Source: CAD feature listing. Evaluate the final solid. Frame: model axes, mm. A direction names the side the tool comes from. Give positions to 0.01 mm unless a question says otherwise; leave off trailing zeros. Loops run counter-clockwise (first coordinate to the right, second up) from the corner with the lowest first, then second, coordinate; pieces in that order, holes last. Notation, with made-up numbers: M 71.25,-29.5 L 101.25,-29.5 A6 cw 101.25,-19.5 Z; hole C 31,88.5 d3. An arc over 180 degrees is marked long. Answer in a Markdown table with one row per item.
```python
from build123d import *

# Parameters (mm, degrees)
BOX005_W        = 20
BOX005_H        = 1
BOX005_DEPTH    = 56
BOX006_W        = 20
BOX006_H        = 1
BOX006_DEPTH    = 56
BOX004_W        = 200
BOX004_H        = 1
BOX004_DEPTH    = 40
BOX002_W        = 1
BOX002_H        = 150
BOX002_DEPTH    = 56
BOX001_W        = 1
BOX001_H        = 150
BOX001_DEPTH    = 56
BOX_W           = 200
BOX_H           = 150
BOX_DEPTH       = 1
BOX003_W        = 200
BOX003_H        = 1
BOX003_DEPTH    = 56
CHAMFER_SIZE    = 2
CHAMFER001_SIZE = 2
CHAMFER002_SIZE = 2
CHAMFER003_SIZE = 2
CHAMFER004_SIZE = 2
CHAMFER005_SIZE = 2


with BuildPart() as cube005:
    # Box005 → Box005 (new body)
    with BuildSketch(Plane.XY):
        with Locations((10, 0.5)):
            Rectangle(BOX005_W, BOX005_H)
    extrude(amount=BOX005_DEPTH)


with BuildPart() as cube006:
    # Box006 → Box006 (new body)
    with BuildSketch(Plane(origin=(180, 0, 0), x_dir=(1, 0, 0), z_dir=(0, 0, 1))):
        with Locations((10, 0.5)):
            Rectangle(BOX006_W, BOX006_H)
    extrude(amount=BOX006_DEPTH)


with BuildPart() as cube004:
    # Box004 → Box004 (new body)
    with BuildSketch(Plane.XY):
        with Locations((100, 0.5)):
            Rectangle(BOX004_W, BOX004_H)
    extrude(amount=BOX004_DEPTH)


with BuildPart() as cube002:
    # Box002 → Box002 (new body)
    with BuildSketch(Plane(origin=(199, 0, 0), x_dir=(1, 0, 0), z_dir=(0, 0, 1))):
        with Locations((0.5, 75)):
            Rectangle(BOX002_W, BOX002_H)
    extrude(amount=BOX002_DEPTH)


with BuildPart() as cube001:
    # Box001 → Box001 (new body)
    with BuildSketch(Plane.XY):
        with Locations((0.5, 75)):
            Rectangle(BOX001_W, BOX001_H)
    extrude(amount=BOX001_DEPTH)


with BuildPart() as cube:
    # Box → Box (new body)
    with BuildSketch(Plane.XY):
        with Locations((100, 75)):
            Rectangle(BOX_W, BOX_H)
    extrude(amount=BOX_DEPTH)


with BuildPart() as fusion005:
    # Box003 → Box003 (new body)
    with BuildSketch(Plane(origin=(0, 149, 0), x_dir=(1, 0, 0), z_dir=(0, 0, 1))):
        with Locations((100, 0.5)):
            Rectangle(BOX003_W, BOX003_H)
    extrude(amount=BOX003_DEPTH)

    # Fusion: union Cube
    add(cube.part)

    # Fusion001: union Cube001
    add(cube001.part)

    # Fusion002: union Cube002
    add(cube002.part)

    # Fusion003: union Cube004
    add(cube004.part)

    # Chamfer
    chamfer_edges = [fusion005.edges().sort_by_distance(p)[0] for p in [
        (100, 149, 1),
    ]]
    chamfer(chamfer_edges, length=CHAMFER_SIZE)

    # Chamfer001
    chamfer001_edges = [fusion005.edges().sort_by_distance(p)[0] for p in [
        (1, 74, 1),
    ]]
    chamfer(chamfer001_edges, length=CHAMFER001_SIZE)

    # Chamfer002
    chamfer002_edges = [fusion005.edges().sort_by_distance(p)[0] for p in [
        (199, 74, 1),
    ]]
    chamfer(chamfer002_edges, length=CHAMFER002_SIZE)

    # Chamfer003
    chamfer003_edges = [fusion005.edges().sort_by_distance(p)[0] for p in [
        (1, 149, 29.5),
    ]]
    chamfer(chamfer003_edges, length=CHAMFER003_SIZE)

    # Chamfer004
    chamfer004_edges = [fusion005.edges().sort_by_distance(p)[0] for p in [
        (199, 149, 29.5),
    ]]
    chamfer(chamfer004_edges, length=CHAMFER004_SIZE)

    # Chamfer005
    chamfer005_edges = [fusion005.edges().sort_by_distance(p)[0] for p in [
        (100, 1, 1),
    ]]
    chamfer(chamfer005_edges, length=CHAMFER005_SIZE)

    # Fusion004: union Cube006
    add(cube006.part)

    # Fusion005: union Cube005
    add(cube005.part)


solid = fusion005.part
```
1) Material intervals for L1, parallel to X at y = 123, z = 10.5; L2, parallel to Y at x = 129.5, z = 18; L3, parallel to Z at x = 18, y = 82.5, sorted ascending.
Reply:
| item | result |
|---|---|
| L1 | x = 0 to 1, 199 to 200 |
| L2 | y = 0 to 1, 149 to 150 |
| L3 | z = 0 to 1 |
2) Pull-direction query (Y, two-part tool) for faces 1 (the flat face through (99, 150, 28)), 2 (the flat face through (99, 0, 21)), 3 (the flat face through (1, 73, 29)), 4 (the flat face through (199, 73, 29)); classes: released by +Y, released by -Y, zero draft, split by the parting line, or undercut.
Reply:
| item | result |
|---|---|
| face 1 | released by +Y |
| face 2 | released by -Y |
| face 3 | undercut |
| face 4 | undercut |
3) Section C-C, the plane z = 10.5. Return loops of the section in (x, y).
Reply:
| item | result |
|---|---|
| outline | M 0,0 L 200,0 L 200,150 L 0,150 Z; hole M 1,1 L 199,1 L 199,147 L 197,149 L 3,149 L 1,147 Z |
4) Section D-D, the plane x = 25.5. Return loops of the section in (y, z), then the cut area to 3 significant figures.
Reply:
| item | result |
|---|---|
| outline | M 0,0 L 150,0 L 150,56 L 149,56 L 149,3 L 147,1 L 3,1 L 1,3 L 1,40 L 0,40 Z |
| area | 248 mm² |
5) Section A-A, the plane y = 62.5. Return loops of the section in (x, z), then the cut area to 3 significant figures.
Reply:
| item | result |
|---|---|
| outline | M 0,0 L 200,0 L 200,56 L 199,56 L 199,3 L 197,1 L 3,1 L 1,3 L 1,56 L 0,56 Z |
| area | 314 mm² |
6) Section B-B, the plane z = 50. Return loops of the section in (x, y).
Reply:
| item | result |
|---|---|
| outline | M 0,0 L 20,0 L 20,1 L 1,1 L 1,147 L 3,149 L 197,149 L 199,147 L 199,1 L 180,1 L 180,0 L 200,0 L 200,150 L 0,150 Z |
7) Pin query (flat end, axial travel): pin 1 Ø12 at (y, z) = (20, 29.5) entering from -X; pin 2 Ø0.5 at (x, y) = (71, 0.5) entering from +Z; pin 3 Ø4 at (x, y) = (138.5, 83.5) entering from +Z. Return the tip coordinate at first contact, or that it passes through.
Reply:
| item | result |
|---|---|
| pin 1 | stops at x = 0 |
| pin 2 | stops at z = 40 |
| pin 3 | stops at z = 1 |
8) Set-up query: faces 5 (the flat face through (200, 74, 28)), 6 (the flat face through (99, 149, 29)). Return all of +Z, -Z, +X, -X, +Y, -Y with unobstructed straight access to the full face (end or side cutting, diameter ignored); none if empty.
Reply:
| item | result |
|---|---|
| face 5 | +Z, -Z, +X, +Y, -Y |
| face 6 | +Z |
